```python
from build123d import *

# Parameters (mm, degrees)
SKETCH1_W           = 120
SKETCH1_H           = 80
BOSS_EXTRUDE1_DEPTH = 33
SKETCH2_W           = 8
SKETCH2_H           = 76
CUT_EXTRUDE1_DEPTH  = 21
SKETCH3_R           = 1.8
CUT_EXTRUDE2_DEPTH  = 76.106590923
SKETCH4_R           = 2.5
CUT_EXTRUDE3_DEPTH  = 106.304320899


with BuildPart() as part:
    # Sketch1 → Boss-Extrude1 (new body)
    with BuildSketch(Plane(origin=(0, 0, 0), x_dir=(1, 0, 0), z_dir=(0, 1, 0))):
        Rectangle(SKETCH1_W, SKETCH1_H)
    extrude(amount=BOSS_EXTRUDE1_DEPTH)

    # Sketch2 → Cut-Extrude1 (cut)
    with BuildSketch(Plane(origin=(0, 33, 0), x_dir=(1, 0, 0), z_dir=(0, 1, 0))):
        with Locations((-56, 2)):
            Rectangle(SKETCH2_W, SKETCH2_H)
    cut_extrude1 = extrude(amount=-CUT_EXTRUDE1_DEPTH, mode=Mode.SUBTRACT)

    # Sketch3 → Cut-Extrude2 (cut, through all)
    with BuildSketch(Plane(origin=(0, 12, 0), x_dir=(1, 0, 0), z_dir=(0, 1, 0))):
        with Locations(Location((-56, 15, 0), (0, 0, 270))):
            Circle(SKETCH3_R)
        with Locations(Location((-56, -12, 0), (0, 0, 270))):
            Circle(SKETCH3_R)
    cut_extrude2 = extrude(amount=-CUT_EXTRUDE2_DEPTH, mode=Mode.SUBTRACT)

    # Sketch4 → Cut-Extrude3 (cut, through all)
    with BuildSketch(Plane.XY.offset(40)):
        with Locations((-54.5, 20.5)):
            Circle(SKETCH4_R)
        with BuildLine():
            Line((-54.5, 23), (-60, 23))
            Line((-60, 23), (-60, 18))
            Line((-60, 18), (-54.5, 18))
            ThreePointArc((-54.5, 18), (-57, 20.5), (-54.5, 23))
        make_face()
    cut_extrude3 = extrude(amount=-CUT_EXTRUDE3_DEPTH, mode=Mode.SUBTRACT)

    # Mirror1: Cut-Extrude1, Cut-Extrude2, Cut-Extrude3 across plane
    add(cut_extrude1.mirror(Plane(origin=(0, 0, 0), x_dir=(0, 0, 1), z_dir=(1, 0, 0))), mode=Mode.SUBTRACT)
    add(cut_extrude2.mirror(Plane(origin=(0, 0, 0), x_dir=(0, 0, 1), z_dir=(1, 0, 0))), mode=Mode.SUBTRACT)
    add(cut_extrude3.mirror(Plane(origin=(0, 0, 0), x_dir=(0, 0, 1), z_dir=(1, 0, 0))), mode=Mode.SUBTRACT)


solid = part.part
```
Build history of the part. All positions in model axes, mm. A direction names the side the tool comes from. Round coordinates to 2 decimals unless told otherwise and drop trailing zeros. Order: outer loops, then holes, each group sorted by start corner. A loop starts at its lowest first (then second) coordinate and runs counter-clockwise, first axis right, second up. Notation, with made-up numbers: (58, 51.5) -> (116, 51.5) arc R11 cw to (116, 67.5) -> close; hole circle Ø10 at (-26, 3). An arc over 180 degrees is marked (long way). Answer in a Markdown table with one row per item.
1) Wall check: L1, parallel to Z at x = 56, y = 3.75; L2, parallel to X at y = 5, z = -15; L3, parallel to X at y = 16.5, z = 19. Give the ranges that are in metal, low to high.
Values:
| item | result |
|---|---|
| L1 | -40 to -16.8, -13.2 to 10.2, 13.8 to 40 |
| L2 | -60 to -57.8, -54.2 to 54.2, 57.8 to 60 |
| L3 | -52 to 52 |
2) Mould opens along Y. For faces 1 (the flat face through (57, 18, 38)), 2 (the flat face through (56, 12, -3)), 3 (the flat face through (-1, 16, -40)) say: released by +Y, released by -Y, zero draft, split by the parting line, or undercut.
Values:
| item | result |
|---|---|
| face 1 | undercut |
| face 2 | released by +Y |
| face 3 | zero draft |
3) Band-saw the part on A-A on z = -15. Give the cut face in (x, y), and give its area (3 significant figures).
Values:
| item | result |
|---|---|
| outline | (-60, 0) -> (-57.8, 0) -> (-57.8, 12) -> (-60, 12) -> close; (-54.2, 0) -> (54.2, 0) -> (54.2, 12) -> (52, 12) -> (52, 33) -> (-52, 33) -> (-52, 12) -> (-54.2, 12) -> close; (57.8, 0) -> (60, 0) -> (60, 12) -> (57.8, 12) -> close |
| area | 3,540 mm2 |
4) Band-saw the part on C-C on z = 28.5. Give the cut face in (x, y).
Values:
| item | result |
|---|---|
| outline | (-60, 0) -> (60, 0) -> (60, 12) -> (52, 12) -> (52, 33) -> (-52, 33) -> (-52, 12) -> (-60, 12) -> close |
5) Pin check, flat tips, straight feed: P1, Ø4, axis at y = 21.5, z = -18, coming from the +X side; P2, Ø4, axis at x = 58, y = 18, coming from the -Z side; P3, Ø4, axis at x = -54.5, z = -0.5, coming from the +Y side. Stop position of each tip, or through.
Values:
| item | result |
|---|---|
| P1 | x = 52 |
| P2 | z = 36 |
| P3 | y = 12 |
6) Band-saw the part on B-B on x = 56. Give the cut face in (y, z).
Values:
| item | result |
|---|---|
| outline | (0, -40) -> (12, -40) -> (12, -16.8) -> (0, -16.8) -> close; (0, -13.2) -> (12, -13.2) -> (12, 10.2) -> (0, 10.2) -> close; (0, 13.8) -> (12, 13.8) -> (12, 36) -> (18, 36) -> (18, 40) -> (0, 40) -> close; (23, 36) -> (33, 36) -> (33, 40) -> (23, 40) -> close |
7) Band-saw the part on D-D on y = 30. Give the cut face in (x, z), and give its area (3 significant figures).
Values:
| item | result |
|---|---|
| outline | (-60, 36) -> (-52, 36) -> (-52, -40) -> (52, -40) -> (52, 36) -> (60, 36) -> (60, 40) -> (-60, 40) -> close |
| area | 8,380 mm2 |
8) Which spindle directions (+Z, -Z, +X, -X, +Y, -Y) get a long thin tool onto all of the face, cutting with end or side? Do faces 4 (the flat face through (60, 7, 1)), 5 (the flat face through (56, 28, 36)), 6 (the flat face through (-56, 15, 36)), 7 (the flat face through (-57, 23, 38)), 8 (the cylindrical face through (57.757, 6.084, -15.39)). Say none if no direction does.
Values:
| item | result |
|---|---|
| face 4 | +Z, -Z, +X, +Y, -Y |
| face 5 | -Z, +X, +Y |
| face 6 | -Z, -X, +Y |
| face 7 | +Z, -Z, -X |
| face 8 | +Y, -Y |
